Read the model definition and answer for the solid it produces. Units are mm, in the model's axes. Coordinates: 2 decimals unless noted, no trailing zeros.
from build123d import *

# Parameters (mm, degrees)
BOSS_EXTRUDE1_DEPTH = 770


with BuildPart() as part:
    # Sketch1 → Boss-Extrude1 (new body)
    with BuildSketch(Plane.XY):
        with BuildLine():
            Line((-14.5, 10), (-14.5, 15))
            Line((-14.5, 15), (-20, 15))
            Line((-20, 15), (-20, -15))
            Line((-20, -15), (-14.5, -15))
            Line((-14.5, -15), (-14.5, -10))
            Line((-14.5, -10), (-11.767766953, -10))
            add(Edge.make_bspline(
                [(-11.767766953, -10), (-10.345177969, -11.422588984), (-8.922588984, -12.845177969), (-7.5, -14.267766953)],
                knots=[0, 0, 0, 0, 1, 1, 1, 1], degree=3))
            Line((-7.5, -14.267766953), (-7.5, -16.653589838))
            Line((-7.5, -16.653589838), (-7.300000072, -16.999999875))
            Line((-7.300000072, -16.999999875), (-7.5, -17.346410162))
            Line((-7.5, -17.346410162), (-7.5, -19.480384758))
            Line((-7.5, -19.480384758), (-7.200000072, -19.999999875))
            Line((-7.200000072, -19.999999875), (-7.5, -20.519615242))
            Line((-7.5, -20.519615242), (-7.5, -22.653589838))
            Line((-7.5, -22.653589838), (-7.3, -23))
            Line((-7.3, -23), (-7.5, -23.346410162))
            Line((-7.5, -23.346410162), (-7.5, -25.732233047))
            add(Edge.make_bspline(
                [(-7.5, -25.732233047), (-8.922588984, -27.154822031), (-10.345177969, -28.577411016), (-11.767766953, -30)],
                knots=[0, 0, 0, 0, 1, 1, 1, 1], degree=3))
            Line((-11.767766953, -30), (-14.5, -30))
            Line((-14.5, -30), (-14.5, -25))
            Line((-14.5, -25), (-20, -25))
            Line((-20, -25), (-20, -37))
            ThreePointArc((-20, -37), (-19.121320344, -39.121320344), (-17, -40))
            Line((-17, -40), (-5, -40))
            Line((-5, -40), (-5, -34.5))
            Line((-5, -34.5), (-10, -34.5))
            Line((-10, -34.5), (-10, -31.767766953))
            add(Edge.make_bspline(
                [(-10, -31.767766953), (-8.577411016, -30.345177969), (-7.154822031, -28.922588984), (-5.732233047, -27.5)],
                knots=[0, 0, 0, 0, 1, 1, 1, 1], degree=3))
            Line((-5.732233047, -27.5), (-3.346410162, -27.5))
            Line((-3.346410162, -27.5), (-3, -27.3))
            Line((-3, -27.3), (-2.653589838, -27.5))
            Line((-2.653589838, -27.5), (-0.519615242, -27.5))
            Line((-0.519615242, -27.5), (-2.17e-07, -27.200000125))
            Line((-2.17e-07, -27.200000125), (0.519615242, -27.5))
            Line((0.519615242, -27.5), (2.653589838, -27.5))
            Line((2.653589838, -27.5), (3, -27.3))
            Line((3, -27.3), (3.346410162, -27.5))
            Line((3.346410162, -27.5), (5.732233047, -27.5))
            add(Edge.make_bspline(
                [(5.732233047, -27.5), (7.154822031, -28.922588984), (8.577411016, -30.345177969), (10, -31.767766953)],
                knots=[0, 0, 0, 0, 1, 1, 1, 1], degree=3))
            Line((10, -31.767766953), (10, -34.5))
            Line((10, -34.5), (5, -34.5))
            Line((5, -34.5), (5, -40))
            Line((5, -40), (17, -40))
            ThreePointArc((17, -40), (19.121320344, -39.121320344), (20, -37))
            Line((20, -37), (20, -25))
            Line((20, -25), (14.5, -25))
            Line((14.5, -25), (14.5, -30))
            Line((14.5, -30), (11.767766953, -30))
            add(Edge.make_bspline(
                [(11.767766953, -30), (10.345177969, -28.577411016), (8.922588984, -27.154822031), (7.5, -25.732233047)],
                knots=[0, 0, 0, 0, 1, 1, 1, 1], degree=3))
            Line((7.5, -25.732233047), (7.5, -23.346410162))
            Line((7.5, -23.346410162), (7.3, -23))
            Line((7.3, -23), (7.5, -22.653589838))
            Line((7.5, -22.653589838), (7.5, -20.519615242))
            Line((7.5, -20.519615242), (7.200000072, -20.000000125))
            Line((7.200000072, -20.000000125), (7.5, -19.480384758))
            Line((7.5, -19.480384758), (7.5, -17.346410162))
            Line((7.5, -17.346410162), (7.300000072, -17.000000125))
            Line((7.300000072, -17.000000125), (7.5, -16.653589838))
            Line((7.5, -16.653589838), (7.5, -14.267766953))
            add(Edge.make_bspline(
                [(7.5, -14.267766953), (8.922588984, -12.845177969), (10.345177969, -11.422588984), (11.767766953, -10)],
                knots=[0, 0, 0, 0, 1, 1, 1, 1], degree=3))
            Line((11.767766953, -10), (14.5, -10))
            Line((14.5, -10), (14.5, -15))
            Line((14.5, -15), (20, -15))
            Line((20, -15), (20, 15))
            Line((20, 15), (14.5, 15))
            Line((14.5, 15), (14.5, 10))
            Line((14.5, 10), (11.767766953, 10))
            add(Edge.make_bspline(
                [(11.767766953, 10), (10.345177969, 11.422588984), (8.922588984, 12.845177969), (7.5, 14.267766953)],
                knots=[0, 0, 0, 0, 1, 1, 1, 1], degree=3))
            Line((7.5, 14.267766953), (7.5, 16.653589838))
            Line((7.5, 16.653589838), (7.300000072, 16.999999875))
            Line((7.300000072, 16.999999875), (7.5, 17.346410162))
            Line((7.5, 17.346410162), (7.5, 19.480384758))
            Line((7.5, 19.480384758), (7.200000072, 19.999999875))
            Line((7.200000072, 19.999999875), (7.5, 20.519615242))
            Line((7.5, 20.519615242), (7.5, 22.653589838))
            Line((7.5, 22.653589838), (7.3, 23))
            Line((7.3, 23), (7.5, 23.346410162))
            Line((7.5, 23.346410162), (7.5, 25.732233047))
            add(Edge.make_bspline(
                [(7.5, 25.732233047), (8.922588984, 27.154822031), (10.345177969, 28.577411016), (11.767766953, 30)],
                knots=[0, 0, 0, 0, 1, 1, 1, 1], degree=3))
            Line((11.767766953, 30), (14.5, 30))
            Line((14.5, 30), (14.5, 25))
            Line((14.5, 25), (20, 25))
            Line((20, 25), (20, 37))
            ThreePointArc((20, 37), (19.121320344, 39.121320344), (17, 40))
            Line((17, 40), (5, 40))
            Line((5, 40), (5, 34.5))
            Line((5, 34.5), (10, 34.5))
            Line((10, 34.5), (10, 31.767766953))
            add(Edge.make_bspline(
                [(10, 31.767766953), (8.577411016, 30.345177969), (7.154822031, 28.922588984), (5.732233047, 27.5)],
                knots=[0, 0, 0, 0, 1, 1, 1, 1], degree=3))
            Line((5.732233047, 27.5), (3.346410162, 27.5))
            Line((3.346410162, 27.5), (3, 27.3))
            Line((3, 27.3), (2.653589838, 27.5))
            Line((2.653589838, 27.5), (0.519615242, 27.5))
            Line((0.519615242, 27.5), (2.17e-07, 27.200000125))
            Line((2.17e-07, 27.200000125), (-0.519615242, 27.5))
            Line((-0.519615242, 27.5), (-2.653589838, 27.5))
            Line((-2.653589838, 27.5), (-3, 27.3))
            Line((-3, 27.3), (-3.346410162, 27.5))
            Line((-3.346410162, 27.5), (-5.732233047, 27.5))
            add(Edge.make_bspline(
                [(-5.732233047, 27.5), (-7.154822031, 28.922588984), (-8.577411016, 30.345177969), (-10, 31.767766953)],
                knots=[0, 0, 0, 0, 1, 1, 1, 1], degree=3))
            Line((-10, 31.767766953), (-10, 34.5))
            Line((-10, 34.5), (-5, 34.5))
            Line((-5, 34.5), (-5, 40))
            Line((-5, 40), (-17, 40))
            ThreePointArc((-17, 40), (-19.121320344, 39.121320344), (-20, 37))
            Line((-20, 37), (-20, 25))
            Line((-20, 25), (-14.5, 25))
            Line((-14.5, 25), (-14.5, 30))
            Line((-14.5, 30), (-11.767766953, 30))
            add(Edge.make_bspline(
                [(-11.767766953, 30), (-10.345177969, 28.577411016), (-8.922588984, 27.154822031), (-7.5, 25.732233047)],
                knots=[0, 0, 0, 0, 1, 1, 1, 1], degree=3))
            Line((-7.5, 25.732233047), (-7.5, 23.346410162))
            Line((-7.5, 23.346410162), (-7.3, 23))
            Line((-7.3, 23), (-7.5, 22.653589838))
            Line((-7.5, 22.653589838), (-7.5, 20.519615242))
            Line((-7.5, 20.519615242), (-7.200000072, 20.000000125))
            Line((-7.200000072, 20.000000125), (-7.5, 19.480384758))
            Line((-7.5, 19.480384758), (-7.5, 17.346410162))
            Line((-7.5, 17.346410162), (-7.300000072, 17.000000125))
            Line((-7.300000072, 17.000000125), (-7.5, 16.653589838))
            Line((-7.5, 16.653589838), (-7.5, 14.267766953))
            add(Edge.make_bspline(
                [(-7.5, 14.267766953), (-8.922588984, 12.845177969), (-10.345177969, 11.422588984), (-11.767766953, 10)],
                knots=[0, 0, 0, 0, 1, 1, 1, 1], degree=3))
            Line((-11.767766953, 10), (-14.5, 10))
        make_face()
        with BuildLine():
            Line((-10.525126266, -7), (-14.5, -7))
            Line((-14.5, -7), (-14.5, 7))
            Line((-14.5, 7), (-10.525126266, 7))
            Line((-10.525126266, 7), (-3.886038516, 13.63908775))
            ThreePointArc((-3.886038516, 13.63908775), (-3.300549454, 15.018813426), (-3.838113574, 16.417907847))
            ThreePointArc((-3.838113574, 16.417907847), (0, 25.25), (3.838113574, 16.417907847))
            ThreePointArc((3.838113574, 16.417907847), (3.300549454, 15.018813426), (3.886038516, 13.63908775))
            add(Edge.make_bspline(
                [(3.886038516, 13.63908775), (6.099067766, 11.4260585), (8.312097016, 9.21302925), (10.525126266, 7)],
                knots=[0, 0, 0, 0, 1, 1, 1, 1], degree=3))
            Line((10.525126266, 7), (14.5, 7))
            Line((14.5, 7), (14.5, -7))
            Line((14.5, -7), (10.525126266, -7))
            add(Edge.make_bspline(
                [(10.525126266, -7), (8.312097016, -9.21302925), (6.099067766, -11.4260585), (3.886038516, -13.63908775)],
                knots=[0, 0, 0, 0, 1, 1, 1, 1], degree=3))
            ThreePointArc((3.886038516, -13.63908775), (3.300549454, -15.018813426), (3.838113574, -16.417907847))
            ThreePointArc((3.838113574, -16.417907847), (0, -25.25), (-3.838113574, -16.417907847))
            ThreePointArc((-3.838113574, -16.417907847), (-3.300549454, -15.018813426), (-3.886038516, -13.63908775))
            add(Edge.make_bspline(
                [(-3.886038516, -13.63908775), (-6.099067766, -11.4260585), (-8.312097016, -9.21302925), (-10.525126266, -7)],
                knots=[0, 0, 0, 0, 1, 1, 1, 1], degree=3))
        make_face(mode=Mode.SUBTRACT)
    extrude(amount=-BOSS_EXTRUDE1_DEPTH)


solid = part.part
Item 1: Determine the mould class of faces 1 (the face through (-14.5, 0, -380)), 2 (the face through (20, 0, -380)), 3 (the face through (14.5, 0, -380)), 4 (the face through (-20, 31, -380)) for opening direction X: released by +X, released by -X, zero draft, split by the parting line, or undercut.
Numbers:
face 1: undercut
face 2: released by +X
face 3: undercut
face 4: released by -X
Item 2: Given pin 1 (2 mm diameter, centred on x = 10, y = 9.5, fed in from +Z); pin 2 (1.7 mm diameter, centred on x = -1.5, z = -498.5, fed in from -Y); pin 3 (2.5 mm diameter, centred on y = -18.5, z = -423.5, fed in from +X); pin 4 (1.6 mm diameter, centred on y = -38.5, z = -404.5, fed in from +X), each flat-ended and moving along its own axis, determine where each tip first touches the part or whether it passes through.
Numbers:
pin 1: stops at z = 0
pin 2: stops at y = -27.5
pin 3: stops at x = 7.5
pin 4: stops at x = 19.92
Item 3: Find the intervals of material crossed by line 1 along X through (y, z) = (14.5, -198.5); line 2 along X through (y, z) = (36, -628); line 3 along Y through (x, z) = (1, -647), in increasing order.
Numbers:
line 1: x = -20 to -14.5, -7.5 to -3.38, 3.38 to 7.5, 14.5 to 20
line 2: x = -20 to -5, 5 to 20
line 3: y = -27.5 to -25.15, 25.15 to 27.5
